Model file for the job. Use its own axes, mm. A direction names the side the tool comes from. Round coordinates to 2 decimals unless told otherwise and drop trailing zeros. Loops run counter-clockwise (first coordinate to the right, second up) from the corner with the lowest first, then second, coordinate; pieces in that order, holes last. Notation, with made-up numbers: M 22.5,48 L 45.5,48 A14 cw 45.5,55 Z; hole C 51,40.5 d11. An arc over 180 degrees is marked long. Use a Markdown table: item, result. Add a question column.
Item 1: Pin check, flat tips, straight feed: P1, Ø3.5, axis at x = 1, y = -14, coming from the -Z side; P2, Ø9, axis at y = 0, z = 15, coming from the +X side; P3, Ø1, axis at x = -5, y = 6, coming from the +Z side. Stop position of each tip, or through.
Item 2: Tool access for faces 4 (the flat face through (0, -15, 15)), 5 (the flat face through (-4.39, 13.52, 14.9)), 6 (the flat face through (-3, 12, 19)), 7 (the flat face through (-5, -14, 25)): list every direction of +Z, -Z, +X, -X, +Y, -Y with a clear straight run to the whole face (end or side of a thin tool).
Item 3: Saw through at A-A on y = 0. Write the cut outline in (x, z).
Item 4: Saw through at D-D on y = -8.25. Write the cut outline in (x, z).
Item 5: Two-plate mould, pull along Y, no slides. Class faces 1 (the flat face through (-12, -8, 16)), 2 (the flat face through (7, -14, 25)), 3 (the flat face through (-4, 15, 18)): +Y half, -Y half, draft (parallel to the pull), parting line (faces both ways), or undercut.
Item 6: Saw through at C-C on x = 4.5. Write the cut outline in (y, z), then the cut area to 3 significant figures.
Item 7: Wall check: L1, parallel to X at y = 11.5, z = 13.75; L2, parallel to Z at x = 13.7, y = 0. Give the ranges that are in metal, low to high. Write a range as from..to.
Item 8: Saw through at B-B on z = 20. Write the cut outline in (x, y), then the cut area to 3 significant figures.
```python
from build123d import *

# Parameters (mm, degrees)
F0_W      = 30
F0_H      = 30
F1_DEPTH  = 30
F2_T      = -3
F3_W      = 15
F3_H      = 15
F4_DEPTH  = 3
F5_R      = 7.5
F6_DEPTH  = 3
F8_DEPTH  = 3
F9_W      = 1
F9_H      = 4
F9_W_2    = 2
F9_W_3    = 3
F9_W_4    = 4
F10_DEPTH = 4


with BuildPart() as f1:
    # F0 (on Top) → F1 (new body)
    with BuildSketch(Plane.XY):
        Rectangle(F0_W, F0_H)
    extrude(amount=F1_DEPTH)

    # F2
    f2_openings = [f1.faces().sort_by_distance(p)[0] for p in [
        (0, 0, 30),
    ]]
    offset(amount=F2_T, openings=f2_openings)

    # F3 (on face) → F4 (cut, through all)
    with BuildSketch(Plane(origin=(-15, 0, 0), x_dir=(0, -1, 0), z_dir=(-1, 0, 0))):
        with Locations((0, 15)):
            Rectangle(F3_W, F3_H)
    extrude(amount=-F4_DEPTH, mode=Mode.SUBTRACT)

    # F5 (on face) → F6 (cut, through all)
    with BuildSketch(Plane.YZ.offset(15)):
        with Locations((0, 15)):
            Circle(F5_R)
    extrude(amount=-F6_DEPTH, mode=Mode.SUBTRACT)

    # F7 (on face) → F8 (cut, through all)
    with BuildSketch(Plane(origin=(0, 15, 0), x_dir=(-1, 0, 0), z_dir=(0, 1, 0))):
        Polygon((8.660254, 7.5), (0, 22.5), (-9.176206, 7.5), align=None)
    extrude(amount=-F8_DEPTH, mode=Mode.SUBTRACT)

    # F9 (on face) → F10 (cut)
    with BuildSketch(Plane.XZ.offset(15)):
        with Locations((-9.5, 27)):
            Rectangle(F9_W, F9_H)
        with Locations((-5, 27)):
            Rectangle(F9_W_2, F9_H)
        with Locations((0.5, 27)):
            Rectangle(F9_W_3, F9_H)
        with Locations((7, 27)):
            Rectangle(F9_W_4, F9_H)
    extrude(amount=-F10_DEPTH, mode=Mode.SUBTRACT)


solid = f1.part
```
Entries:
| question | item | result |
|---|---|---|
| 1 | P1 | z = 0 |
| 1 | P2 | through |
| 1 | P3 | z = 3 |
| 2 | face 4 | +Z, -Z, +X, -X, -Y |
| 2 | face 5 | +Y |
| 2 | face 6 | +Z |
| 2 | face 7 | -Y |
| 3 | outline | M -15,0 L 15,0 L 15,7.5 L 12,7.5 L 12,3 L -12,3 L -12,7.5 L -15,7.5 Z; M -15,22.5 L -12,22.5 L -12,30 L -15,30 Z; M 12,22.5 L 15,22.5 L 15,30 L 12,30 Z |
| 4 | outline | M -15,0 L 15,0 L 15,30 L 12,30 L 12,3 L -12,3 L -12,30 L -15,30 Z |
| 5 | face 1 | undercut |
| 5 | face 2 | draft |
| 5 | face 3 | +Y half |
| 6 | outline | M -15,0 L 15,0 L 15,7.5 L 12,7.5 L 12,3 L -12,3 L -12,30 L -15,30 Z; M 12,15.14 L 15,15.14 L 15,30 L 12,30 Z |
| 6 | area | 229 mm2 |
| 7 | L1 | -15..-12, 12..15 |
| 7 | L2 | 0..7.5, 22.5..30 |
| 8 | outline | M -15,-15 L 15,-15 L 15,-5.59 L 12,-5.59 L 12,-12 L -12,-12 L -12,-7.5 L -15,-7.5 Z; M -15,7.5 L -12,7.5 L -12,12 L -1.44,12 L -1.44,15 L -15,15 Z; M 1.53,12 L 12,12 L 12,5.59 L 15,5.59 L 15,15 L 1.53,15 Z |
| 8 | area | 237 mm2 |
